The listing builds one solid part. Answer for the finished solid, in the listing's coordinates (mm). Face numbers are marked on the shaded views. A direction names the side the tool comes from. Round coordinates to 2 decimals unless told otherwise and drop trailing zeros. Order: outer loops, then holes, each group sorted by start corner. A loop starts at its lowest first (then second) coordinate and runs counter-clockwise, first axis right, second up. Notation, with made-up numbers: M -8,-12.75 L -3,-12.75 A14 cw -3,1.25 Z; hole C 80.25,-37 d11. An arc over 180 degrees is marked long. Write item = value, one per line. Start each with the question number.
(1) A cutting plane is placed at C-C, the plane y = 15.2. Count the separate pieces of the cut face and the enclosed holes in it, and give its area (3 significant figures).
(2) A cutting plane is placed at B-B, the plane z = -29.5. Determine the outline of the cut face in (x, y).
(3) For a pull along Y with two mould halves and no side action, classify the marked faces 1, 2 and 3 as released by +Y, released by -Y, zero draft, split by the parting line, or undercut.
(4) Which of the six approach directions +Z, -Z, +X, -X, +Y, -Y give full straight-line access (tool end or side, diameter ignored) to the marked faces 4, 5 and 6?
(5) A cutting plane is placed at A-A, the plane y = 6.7. Determine the outline of the cut face in (x, z).
(6) A cutting plane is placed at D-D, the plane z = -10. Determine the outline of the cut face in (x, y), and give its area (3 significant figures).
(7) Each of these flat-tipped pins is pushed along its axis until it touches: pin 1 (11.5 mm diameter, centred on x = 10, z = -10, fed in from +Y); pin 2 (6.5 mm diameter, centred on x = 10, y = 21.7, fed in from +Z); pin 3 (3.5 mm diameter, centred on y = -6.5, z = -8, fed in from +X); pin 4 (8 mm diameter, centred on y = 2, z = -48.5, fed in from -X). Where does it stop, or does it pass through?
(8) Straight lines are drawn through the part: probe 1 along Z at (x, y) = (-24, 28); probe 2 along Y at (x, z) = (-10, -26); probe 3 along X at (y, z) = (28, -5). For each, find the intervals that lie inside material, in ascending order. Write a range as from..to.
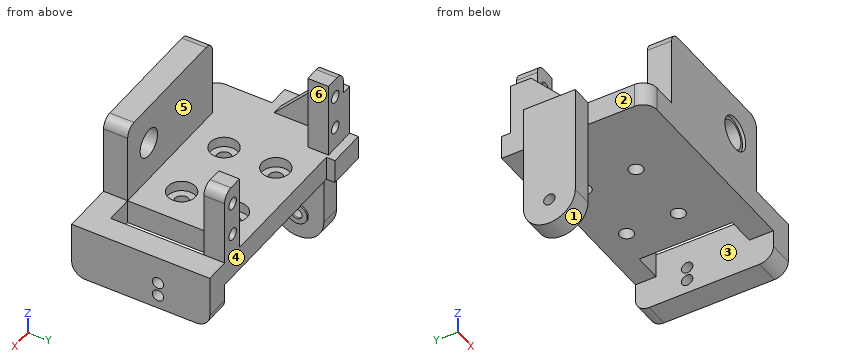
from build123d import *

# Parameters (mm, degrees)
EXTRUDE_START       = 24.2
SKETCH_4_R          = 1.75
EXTRUDE_1_DEPTH     = 6
SKETCH_5_W          = 40
SKETCH_5_H          = 34
SKETCH_5_R          = 2
EXTRUDE_2_DEPTH     = 7
CUT_EXTRUDE_START   = -21.5
SKETCH_6_R          = 4
CUT_EXTRUDE_1_DEPTH = 3
EXTRUDE_START_2     = -9.8
SKETCH_7_R          = 4.1
EXTRUDE_3_DEPTH     = 7
SKETCH_8_R          = 4.9
CUT_EXTRUDE_2_DEPTH = 0.9
EXTRUDE_START_3     = -53
SKETCH_9_R          = 1.65
EXTRUDE_4_DEPTH     = 6
EXTRUDE_START_4     = -21.5
EXTRUDE_5_DEPTH     = 7
EXTRUDE_START_5     = -28
EXTRUDE_7_DEPTH     = 3
EXTRUDE_START_6     = 28
SKETCH_14_R         = 1.65
EXTRUDE_8_DEPTH     = 7
SKETCH_15_W         = 8
SKETCH_15_H         = 7
EXTRUDE_9_DEPTH     = 7
SKETCH_17_R         = 3
SKETCH_17_R_2       = 1.5
EXTRUDE_11_DEPTH    = 0.5


with BuildPart() as part:
    # Sketch 4 → Extrude 1 (new body)
    with BuildSketch(Plane(origin=(0, 0, 0), x_dir=(1, 0, 0), z_dir=(0, 1, 0)).offset(EXTRUDE_START)):
        with BuildLine():
            Line((-28, 28.5), (28, 28.5))
            Line((28, 28.5), (28, 2.5))
            ThreePointArc((28, 2.5), (27.121320344, 0.378679656), (25, -0.5))
            Line((25, -0.5), (21, -0.5))
            Line((21, -0.5), (21, 21.5))
            Line((21, 21.5), (-21, 21.5))
            Line((-21, 21.5), (-21, -0.5))
            Line((-21, -0.5), (-25, -0.5))
            ThreePointArc((-25, -0.5), (-27.121320344, 0.378679656), (-28, 2.5))
            Line((-28, 2.5), (-28, 28.5))
        make_face()
        with Locations(Location((-24.2, 14.9, 0), (0, 0, 90))):
            Circle(SKETCH_4_R, mode=Mode.SUBTRACT)
        with Locations(Location((-24.2, 5.1, 0), (0, 0, 90))):
            Circle(SKETCH_4_R, mode=Mode.SUBTRACT)
        with Locations(Location((24.2, 14.9, 0), (0, 0, 90))):
            Circle(SKETCH_4_R, mode=Mode.SUBTRACT)
        with Locations(Location((24.2, 5.1, 0), (0, 0, 90))):
            Circle(SKETCH_4_R, mode=Mode.SUBTRACT)
    extrude(amount=EXTRUDE_1_DEPTH)

    # Sketch 5 → Extrude 2 (add)
    with BuildSketch(Plane(origin=(0, 0, -28.5), x_dir=(-1, 0, 0), z_dir=(0, 0, -1))):
        with Locations((0, 7.2)):
            Rectangle(SKETCH_5_W, SKETCH_5_H)
        with Locations((-10, 21.7)):
            Circle(SKETCH_5_R, mode=Mode.SUBTRACT)
        with Locations(Location((10, 21.7, 0), (0, 0, 180))):
            Circle(SKETCH_5_R, mode=Mode.SUBTRACT)
        with Locations((10, 6.7)):
            Circle(SKETCH_5_R, mode=Mode.SUBTRACT)
        with Locations(Location((-10, 6.7, 0), (0, 0, 180))):
            Circle(SKETCH_5_R, mode=Mode.SUBTRACT)
    extrude(amount=-EXTRUDE_2_DEPTH)

    # Sketch 6 → Cut-Extrude 1 (cut)
    with BuildSketch(Plane.XY.offset(CUT_EXTRUDE_START)):
        with Locations((-10, 21.7)):
            Circle(SKETCH_6_R)
        with Locations((10, 21.7)):
            Circle(SKETCH_6_R)
        with Locations((-10, 6.7)):
            Circle(SKETCH_6_R)
        with Locations((10, 6.7)):
            Circle(SKETCH_6_R)
    extrude(amount=-CUT_EXTRUDE_1_DEPTH, mode=Mode.SUBTRACT)

    # Sketch 7 → Extrude 3 (add)
    with BuildSketch(Plane(origin=(0, 0, 0), x_dir=(1, 0, 0), z_dir=(0, 1, 0)).offset(EXTRUDE_START_2)):
        with BuildLine():
            Line((20, 21.5), (-20, 21.5))
            Line((-20, 21.5), (-20, 1.5))
            ThreePointArc((-20, 1.5), (-19.121320344, -0.621320344), (-17, -1.5))
            Line((-17, -1.5), (17, -1.5))
            ThreePointArc((17, -1.5), (19.121320344, -0.621320344), (20, 1.5))
            Line((20, 1.5), (20, 21.5))
        make_face()
        with Locations(Location((10, 10, 0), (0, 0, 90))):
            Circle(SKETCH_7_R, mode=Mode.SUBTRACT)
    extrude(amount=EXTRUDE_3_DEPTH)

    # Sketch 8 → Cut-Extrude 2 (cut)
    with BuildSketch(Plane.XZ.offset(9.8)):
        with Locations(Location((10, -10, 0), (0, 0, 270))):
            Circle(SKETCH_8_R)
    extrude(amount=-CUT_EXTRUDE_2_DEPTH, mode=Mode.SUBTRACT)



with BuildPart() as body_2:
    # Sketch 9 → Extrude 4 (new body)
    with BuildSketch(Plane(origin=(22, 25.2, -45.868265324), x_dir=(0, 0, 1), z_dir=(1, 0, 0)).offset(EXTRUDE_START_3)):
        with BuildLine():
            Line((-7.631734676, 2.5), (24.368265324, 2.5))
            Line((24.368265324, 2.5), (24.368265324, 17.5))
            Line((24.368265324, 17.5), (-7.631734676, 17.5))
            ThreePointArc((-7.631734676, 17.5), (-15.131734676, 10), (-7.631734676, 2.5))
        make_face()
        with Locations(Location((-7.631734676, 10, 0), (0, 0, 180))):
            Circle(SKETCH_9_R, mode=Mode.SUBTRACT)
    extrude(amount=-EXTRUDE_4_DEPTH)


with BuildPart() as part_1:
    add(part.part)

    add(body_2.part)  # Extrude 5 merges body 2
    # Sketch 10 → Extrude 5 (add)
    with BuildSketch(Plane.XY.offset(EXTRUDE_START_4)):
        with BuildLine():
            Line((-31, 32.7), (-20, 32.7))
            Line((-20, 32.7), (-20, -9.8))
            Line((-20, -9.8), (-27, -9.8))
            ThreePointArc((-27, -9.8), (-29.828427125, -8.628427125), (-31, -5.8))
            Line((-31, -5.8), (-31, 32.7))
        make_face()
    extrude(amount=-EXTRUDE_5_DEPTH)

    # Sketch 12 → Extrude 7 (add)
    with BuildSketch(Plane(origin=(0, 0, 0), x_dir=(0, 0, -1), z_dir=(1, 0, 0)).offset(EXTRUDE_START_5)):
        Polygon((6.5, 30.2), (6.5, 24.2), (21.5, 10.2), (21.5, 30.2), align=None)
    extrude(amount=-EXTRUDE_7_DEPTH)

    # Sketch 14 → Extrude 8 (add)
    with BuildSketch(Plane(origin=(0, 0, 0), x_dir=(0, 0, -1), z_dir=(1, 0, 0)).offset(EXTRUDE_START_6)):
        with BuildLine():
            Line((21.5, 30.2), (33.5, 30.2))
            ThreePointArc((33.5, 30.2), (36.328427125, 29.028427125), (37.5, 26.2))
            Line((37.5, 26.2), (37.5, -5.8))
            ThreePointArc((37.5, -5.8), (36.328427125, -8.628427125), (33.5, -9.8))
            Line((33.5, -9.8), (21.5, -9.8))
            Line((21.5, -9.8), (21.5, 30.2))
        make_face()
        with Locations((29.5, 15.2)):
            Circle(SKETCH_14_R, mode=Mode.SUBTRACT)
        with Locations((33.5, 15.2)):
            Circle(SKETCH_14_R, mode=Mode.SUBTRACT)
    extrude(amount=EXTRUDE_8_DEPTH)

    # Sketch 15 → Extrude 9 (add)
    with BuildSketch(Plane(origin=(0, 0, 0), x_dir=(1, 0, 0), z_dir=(0, 1, 0)).offset(EXTRUDE_START_2)):
        with Locations((24, 25)):
            Rectangle(SKETCH_15_W, SKETCH_15_H)
    extrude(amount=EXTRUDE_9_DEPTH)

    # Sketch 17 → Extrude 11 (add)
    with BuildSketch(Plane(origin=(-31, 0, 0), x_dir=(0, 0, -1), z_dir=(1, 0, 0))):
        with Locations(Location((53.5, 15.2, 0), (0, 0, 90))):
            Circle(SKETCH_17_R)
        with Locations(Location((53.5, 15.2, 0), (0, 0, 90))):
            Circle(SKETCH_17_R_2, mode=Mode.SUBTRACT)
    extrude(amount=EXTRUDE_11_DEPTH)


solid = part_1.part
Reported:
q1.separate_pieces = 5
q1.enclosed_holes = 0
q1.area = 658 mm²
q2.outline = M -37,7.7 L -31,7.7 L -31,22.7 L -37,22.7 Z; M 28,-9.8 L 35,-9.8 L 35,13.55 L 28,13.55 Z; M 28,16.85 L 35,16.85 L 35,30.2 L 28,30.2 Z
q3.face_1 = split by the parting line
q3.face_2 = zero draft
q3.face_3 = undercut
q4.face_4 = +Z, -Z, +X, +Y
q4.face_5 = +Z, +X, -X, +Y
q4.face_6 = +Z, +Y, -Y
q5.outline = M -31,-28.5 L -12,-28.5 L -12,-24.5 L -14,-24.5 L -14,-21.5 L -31,-21.5 Z; M -8,-28.5 L 8,-28.5 L 8,-24.5 L 6,-24.5 L 6,-21.5 L -6,-21.5 L -6,-24.5 L -8,-24.5 Z; M 12,-28.5 L 20,-28.5 L 20,-21.5 L 14,-21.5 L 14,-24.5 L 12,-24.5 Z; M 28,-37.5 L 35,-37.5 L 35,-21.5 L 28,-21.5 Z
q6.outline = M -31,20.93 L -28,20.93 L -28,24.2 L -21,24.2 L -21,30.2 L -31,30.2 Z; M -20,-9.8 L 5.1,-9.8 L 5.1,-8.9 L 5.9,-8.9 L 5.9,-2.8 L -20,-2.8 Z; M 14.1,-8.9 L 14.9,-8.9 L 14.9,-9.8 L 20,-9.8 L 20,-2.8 L 14.1,-2.8 Z; M 21,24.2 L 28,24.2 L 28,30.2 L 21,30.2 Z
q6.area = 333 mm²
q7.pin_1 = -2.8
q7.pin_2 = -24.5
q7.pin_3 = 20
q7.pin_4 = through
q8.probe_1 = -28.5..-16.64, -13.16..-6.84, -3.36..0.5
q8.probe_2 = -9.8..4.7, 8.7..19.7, 23.7..30.2
q8.probe_3 = -28..-25.95, -22.45..-21, 21..22.45, 25.95..28
